Here's how the part is built. I have some questions about the finished solid (model axes, mm). A direction names the side the tool comes from. Give positions to 0.01 mm unless a question says otherwise; leave off trailing zeros. Order: outer loops, then holes, each group sorted by start corner. A loop starts at its lowest first (then second) coordinate and runs counter-clockwise, first axis right, second up. Notation, with made-up numbers: (51, 2) - (87, 2) arc R13 cw to (87, 23) - close; hole circle Ø11 at (49.5, -2.75). An arc over 180 degrees is marked (long way). One line per question, with ' | ' between items.
from build123d import *

# Parameters (mm, degrees)
SKETCH049_W     = 118.6
SKETCH049_H     = 67
PAD008_DEPTH    = 2
SKETCH050_R     = 1.6
POCKET017_DEPTH = 2
CHAMFER001_SIZE = 1.6
PAD018_DEPTH    = 0.4
POCKET023_DEPTH = 2.401


with BuildPart() as part:
    # Sketch049 → Pad008 (new body)
    with BuildSketch(Plane.XY):
        with Locations((0, -40.1)):
            Rectangle(SKETCH049_W, SKETCH049_H)
    extrude(amount=-PAD008_DEPTH)

    # Sketch050 (on Face5 of Pad008) → Pocket017 (cut)
    with BuildSketch(Plane.XY):
        with Locations((0, -11.6)):
            Circle(SKETCH050_R)
        with Locations((54.3, -40.1)):
            Circle(SKETCH050_R)
        with Locations((-54.3, -40.1)):
            Circle(SKETCH050_R)
        with Locations((0, -68.6)):
            Circle(SKETCH050_R)
    extrude(amount=-POCKET017_DEPTH, mode=Mode.SUBTRACT)

    # Chamfer001
    chamfer001_edges = [part.edges().sort_by_distance(p)[0] for p in [
        (-55.9, -40.1, 0),
        (-1.6, -11.6, 0),
        (52.7, -40.1, 0),
        (-1.6, -68.6, 0),
    ]]
    chamfer(chamfer001_edges, length=CHAMFER001_SIZE)

    # Sketch052 (on Face11 of Chamfer001) → Pad018 (join)
    with BuildSketch(Plane(origin=(0, 0, -2), x_dir=(1, 0, 0), z_dir=(0, 0, -1))):
        Polygon((-59.3, 73.6), (-3.4, 73.6), (-3.4, 71.6), (-57.3, 71.6), (-57.3, 43.5), (-59.3, 43.5), align=None)
        Polygon((59.3, 73.6), (3.4, 73.6), (3.4, 71.6), (57.3, 71.6), (57.3, 43.5), (59.3, 43.5), align=None)
        Polygon((59.3, 6.6), (3.4, 6.6), (3.4, 8.6), (57.3, 8.6), (57.3, 36.7), (59.3, 36.7), align=None)
        Polygon((-59.3, 6.6), (-3.4, 6.6), (-3.4, 8.6), (-57.3, 8.6), (-57.3, 36.7), (-59.3, 36.7), align=None)
    extrude(amount=PAD018_DEPTH)

    # Sketch065 (on Face1 of Pad018) → Pocket023 (cut, through all)
    with BuildSketch(Plane.XY):
        with BuildLine():
            ThreePointArc((-48.8, -11.4), (-49.8, -12.4), (-48.8, -13.4))
            Line((-48.8, -13.4), (-43.8, -13.4))
            ThreePointArc((-43.8, -13.4), (-42.8, -12.4), (-43.8, -11.4))
            Line((-48.8, -11.4), (-43.8, -11.4))
        make_face()
        with BuildLine():
            ThreePointArc((-52.3, -15.4), (-53.3, -16.4), (-52.3, -17.4))
            Line((-52.3, -17.4), (-40.3, -17.4))
            ThreePointArc((-40.3, -17.4), (-39.3, -16.4), (-40.3, -15.4))
            Line((-52.3, -15.4), (-40.3, -15.4))
        make_face()
        with BuildLine():
            ThreePointArc((-48.8, -19.4), (-49.8, -20.4), (-48.8, -21.4))
            Line((-48.8, -21.4), (-43.8, -21.4))
            ThreePointArc((-43.8, -21.4), (-42.8, -20.4), (-43.8, -19.4))
            Line((-48.8, -19.4), (-43.8, -19.4))
        make_face()
        Polygon((-17.7, -32.8), (-7.7, -32.8), (-2.7, -37.8), (-7.7, -42.8), (-17.7, -42.8), align=None)
        Polygon((-5, -20.1), (5, -20.1), (5, -30.1), (0, -35.1), (-5, -30.1), align=None)
        Polygon((7.7, -32.8), (17.7, -32.8), (17.7, -42.8), (7.7, -42.8), (2.7, -37.8), align=None)
        Polygon((5, -45.9), (5, -55.9), (-5, -55.9), (-5, -45.9), (0, -40.9), align=None)
    extrude(amount=-POCKET023_DEPTH, mode=Mode.SUBTRACT)


solid = part.part
1) I want a section at C-C (x = -23.5). List the corners of the cut face in (y, z) for me, plus the area to 3 significant figures.
Model answer:
outline: (-73.6, -2.4) - (-71.6, -2.4) - (-71.6, -2) - (-8.6, -2) - (-8.6, -2.4) - (-6.6, -2.4) - (-6.6, 0) - (-73.6, 0) - close | area: 136 mm2
2) I'm going to push a flat-ended pin straight in: P1, Ø4, axis at x = 0, y = -68.6, coming from the -Z side. Where does the tip first touch, or does it pass through?
Model answer:
P1: stops at z = -2
3) Thinking about a two-plate mould opening in Y: for faces 3 (the face through (-1, -73.6, -1)), 4 (the face through (-2.5, -43.4, -1)), 5 (the face through (-1, -40, 0)), which applies, +Y half, -Y half, draft (parallel to the pull), parting line (faces both ways), or undercut?
Model answer:
face 3: -Y half | face 4: undercut | face 5: draft
4) I want a section at A-A (x = 54.3). List the corners of the cut face in (y, z) for me, plus the area to 3 significant figures.
Model answer:
outline: (-73.6, -2.4) - (-71.6, -2.4) - (-71.6, -2) - (-41.7, -2) - (-41.7, -1.6) - (-43.3, 0) - (-73.6, 0) - close; (-38.5, -2) - (-8.6, -2) - (-8.6, -2.4) - (-6.6, -2.4) - (-6.6, 0) - (-36.9, 0) - (-38.5, -1.6) - close | area: 127 mm2
5) I want a section at D-D (y = -68.6). List the corners of the cut face in (x, z) for me, plus the area to 3 significant figures.
Model answer:
outline: (-59.3, -2.4) - (-57.3, -2.4) - (-57.3, -2) - (-1.6, -2) - (-1.6, -1.6) - (-3.2, 0) - (-59.3, 0) - close; (1.6, -2) - (57.3, -2) - (57.3, -2.4) - (59.3, -2.4) - (59.3, 0) - (3.2, 0) - (1.6, -1.6) - close | area: 230 mm2
6) Please list where these lines run through material, in increasing order: L1, parallel to X at y = -35.5, z = -0.8; L2, parallel to Y at x = 0, z = -1.7; L3, parallel to Y at x = -52, z = -1.85.
Model answer:
L1: x = -59.3 to -17.7, -5 to 5, 17.7 to 59.3 | L2: y = -73.6 to -70.2, -67 to -55.9, -40.9 to -35.1, -20.1 to -13.2, -10 to -6.6 | L3: y = -73.6 to -17.4, -15.4 to -6.6
7) I want a section at B-B (y = -54). List the corners of the cut face in (x, z) for me.
Model answer:
outline: (-59.3, -2.4) - (-57.3, -2.4) - (-57.3, -2) - (-5, -2) - (-5, 0) - (-59.3, 0) - close; (5, -2) - (57.3, -2) - (57.3, -2.4) - (59.3, -2.4) - (59.3, 0) - (5, 0) - close
8) On a 3-axis mill with a long thin cutter (end or side, diameter ignored), from which of +Z, -Z, +X, -X, +Y, -Y can I reach the whole of each face in a straight line? I mean faces 1 (the face through (-5.2, -40.3, -1)), 2 (the face through (59.3, -41, -1)). Say none if no direction works.
Model answer:
face 1: +Z, -Z | face 2: +Z, -Z, +X, +Y, -Y
